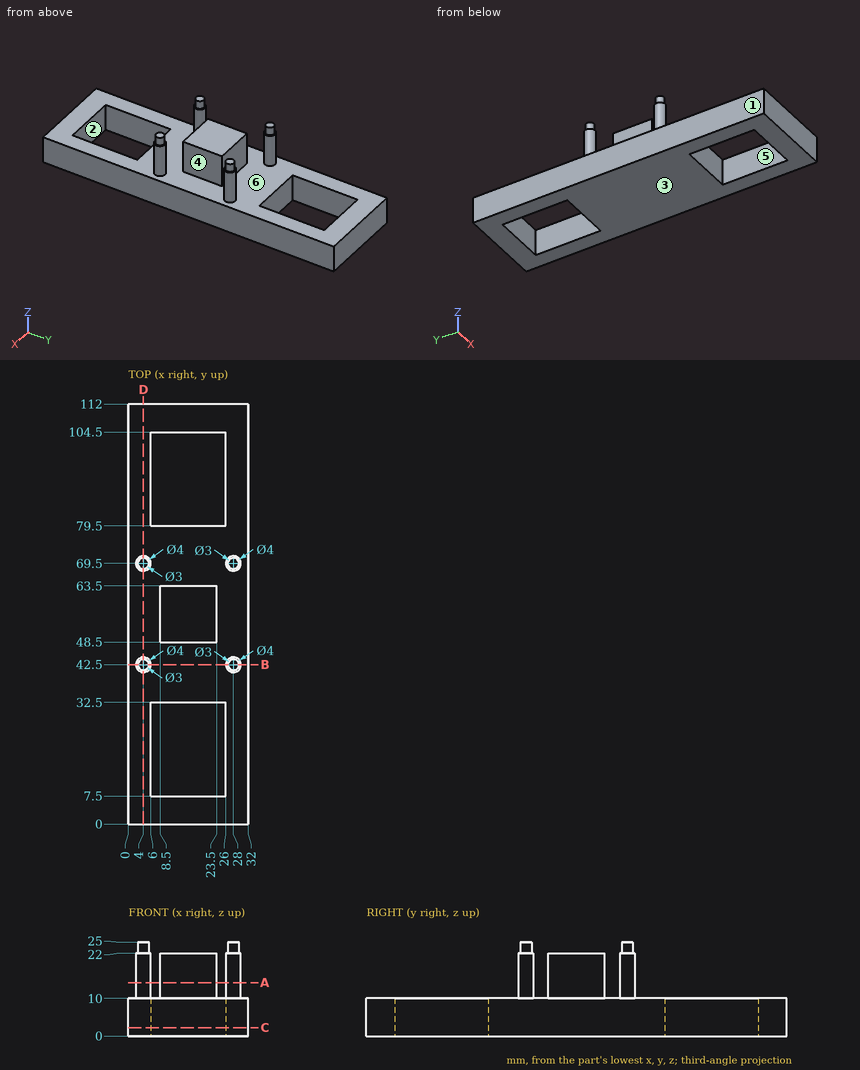
Can you work these out from the drawing? Everything is in mm from the part's minimum corner. A direction names the side the tool comes from. Coordinates: 2 decimals unless noted, no trailing zeros. Loops run counter-clockwise (first coordinate to the right, second up) from the corner with the lowest first, then second, coordinate; pieces in that order, holes last. Notation, with made-up numbers: M -35,-31 L -14,-31 A18 cw -14,-9 Z; hole C 71,-40 d3. An arc over 180 degrees is marked long. One line per item, written item: value.
1. Imagine slicing it at B-B (y = 42.5). List the corners of the cut face in (x, z) for me, and give its area (3 significant figures).
Geometry says:
outline: M 0,0 L 32,0 L 32,10 L 30,10 L 30,22 L 29.5,22 L 29.5,25 L 26.5,25 L 26.5,22 L 26,22 L 26,10 L 6,10 L 6,22 L 5.5,22 L 5.5,25 L 2.5,25 L 2.5,22 L 2,22 L 2,10 L 0,10 Z
area: 434 mm2
2. Imagine slicing it at C-C (z = 2.25). List the corners of the cut face in (x, y) for me, and give its area (3 significant figures).
Geometry says:
outline: M 0,0 L 32,0 L 32,112 L 0,112 Z; hole M 6,7.5 L 26,7.5 L 26,32.5 L 6,32.5 Z; hole M 6,79.5 L 26,79.5 L 26,104.5 L 6,104.5 Z
area: 2,580 mm2
3. Thinking about a two-plate mould opening in X: for the marked faces 1, 2 and 3, which applies, +X half, -X half, draft (parallel to the pull), parting line (faces both ways), or undercut?
Geometry says:
face 1: -X half
face 2: undercut
face 3: draft
4. On a 3-axis mill with a long thin cutter (end or side, diameter ignored), from which of +Z, -Z, +X, -X, +Y, -Y can I reach the whole of each face in a straight line? I mean the marked faces 4, 5 and 6. Say none if no direction works.
Geometry says:
face 4: +Z, +X, +Y, -Y
face 5: +Z, -Z
face 6: +Z
5. Imagine slicing it at A-A (z = 14.25). List the corners of the cut face in (x, y) for me, and give its area (3 significant figures).
Geometry says:
outline: C 4,42.5 d4; C 4,69.5 d4; M 8.5,48.5 L 23.5,48.5 L 23.5,63.5 L 8.5,63.5 Z; C 28,42.5 d4; C 28,69.5 d4
area: 275 mm2
6. Imagine slicing it at D-D (x = 4). List the corners of the cut face in (y, z) for me, and give its area (3 significant figures).
Geometry says:
outline: M 0,0 L 112,0 L 112,10 L 71.5,10 L 71.5,22 L 71,22 L 71,25 L 68,25 L 68,22 L 67.5,22 L 67.5,10 L 44.5,10 L 44.5,22 L 44,22 L 44,25 L 41,25 L 41,22 L 40.5,22 L 40.5,10 L 0,10 Z
area: 1,230 mm2
7. Please list where these lines run through material, in increasing order: probe 1 along Y at (x, z) = (11, 5.75); probe 2 along X at (y, z) = (101.5, 8); probe 3 along Z at (x, y) = (12, 72).
Geometry says:
probe 1: y = 0 to 7.5, 32.5 to 79.5, 104.5 to 112
probe 2: x = 0 to 6, 26 to 32
probe 3: z = 0 to 10
8. Will these pins go through, and if not, where does the flat tip stop? pin 1 Ø1.5 at (x, y) = (11, 61.5) entering from -Z; pin 2 Ø8 at (x, y) = (15, 58.5) entering from +Z; pin 3 Ø9.5 at (y, z) = (55.5, 17) entering from +X; pin 4 Ø12 at (x, y) = (17, 38) entering from +Z.
Geometry says:
pin 1: stops at z = 0
pin 2: stops at z = 22
pin 3: stops at x = 23.5
pin 4: stops at z = 10
